```python
from build123d import *

# Parameters (mm, degrees)
RESSALTO_EXTRUS_O1_DEPTH = 59
ESBO_O2_W                = 50
ESBO_O2_H                = 43.8
CORTE_EXTRUS_O1_DEPTH    = 49
ESBO_O3_R                = 1.75
CORTE_EXTRUS_O2_DEPTH    = 92.553263186
ESBO_O4_W                = 5.65
ESBO_O4_H                = 50
ESBO_O4_R                = 1.75
RESSALTO_EXTRUS_O2_DEPTH = 1
ESBO_O5_R                = 4.35
CORTE_EXTRUS_O3_DEPTH    = 4
ESBO_O6_R                = 11.5
ESBO_O6_R_2              = 1.6
ESBO_O6_R_3              = 4.1
CORTE_EXTRUS_O4_DEPTH    = 6.2
ESBO_O7_W                = 146.645029728
ESBO_O7_H                = 95.479941405
CORTE_EXTRUS_O5_DEPTH    = 139


with BuildPart() as part:
    # Esboço1 → Ressalto-extrusão1 (new body)
    with BuildSketch(Plane.XY):
        Polygon((9, 0), (58, 43.8), (58, 50), (0, 50), (0, 0), align=None)
    extrude(amount=RESSALTO_EXTRUS_O1_DEPTH)

    # Esboço2 → Corte-extrusão1 (cut)
    with BuildSketch(Plane(origin=(58, 0, 0), x_dir=(0, 0, -1), z_dir=(1, 0, 0))):
        with Locations((-29, 21.9)):
            Rectangle(ESBO_O2_W, ESBO_O2_H)
    extrude(amount=-CORTE_EXTRUS_O1_DEPTH, mode=Mode.SUBTRACT)

    # Esboço3 → Corte-extrusão2 (cut, through all)
    with BuildSketch(Plane(origin=(9, 0, 0), x_dir=(0, 0, -1), z_dir=(1, 0, 0))):
        with Locations((-29, 11.9)):
            Circle(ESBO_O3_R)
        with Locations((-29, 31.9)):
            Circle(ESBO_O3_R)
        with Locations((-9, 31.9)):
            Circle(ESBO_O3_R)
        with Locations((-9, 11.9)):
            Circle(ESBO_O3_R)
    extrude(amount=-CORTE_EXTRUS_O2_DEPTH, mode=Mode.SUBTRACT)

    # Esboço4 → Ressalto-extrusão2 (add)
    # profile 1 of 2: a face of its own
    with BuildSketch(Plane.ZY):
        with Locations((9, 25)):
            Rectangle(ESBO_O4_W, ESBO_O4_H)
        with Locations(Location((9, 11.9, 0), (0, 0, 180))):
            Circle(ESBO_O4_R, mode=Mode.SUBTRACT)
        with Locations(Location((9, 31.9, 0), (0, 0, 180))):
            Circle(ESBO_O4_R, mode=Mode.SUBTRACT)
    # profile 2 of 2: a face of its own
    with BuildSketch(Plane.ZY):
        with Locations((29, 25)):
            Rectangle(ESBO_O4_W, ESBO_O4_H)
        with Locations(Location((29, 11.9, 0), (0, 0, 180))):
            Circle(ESBO_O4_R, mode=Mode.SUBTRACT)
        with Locations(Location((29, 31.9, 0), (0, 0, 180))):
            Circle(ESBO_O4_R, mode=Mode.SUBTRACT)
    extrude(amount=RESSALTO_EXTRUS_O2_DEPTH)

    # Esboço5 → Corte-extrusão3 (cut)
    with BuildSketch(Plane(origin=(9, 0, 0), x_dir=(0, 0, -1), z_dir=(1, 0, 0))):
        with Locations((-29, 31.9)):
            Circle(ESBO_O5_R)
        with Locations((-9, 31.9)):
            Circle(ESBO_O5_R)
        with Locations((-29, 11.9)):
            Circle(ESBO_O5_R)
        with Locations((-9, 11.9)):
            Circle(ESBO_O5_R)
    extrude(amount=-CORTE_EXTRUS_O3_DEPTH, mode=Mode.SUBTRACT)

    # Esboço6 → Corte-extrusão4 (cut)
    with BuildSketch(Plane(origin=(0, 50, 0), x_dir=(1, 0, 0), z_dir=(0, 1, 0))):
        with Locations(Location((37, -29, 0), (0, 0, 270))):
            Circle(ESBO_O6_R)
        with Locations(Location((21.5, -13.5, 0), (0, 0, 270))):
            Circle(ESBO_O6_R_2)
        with Locations(Location((52.5, -13.5, 0), (0, 0, 270))):
            Circle(ESBO_O6_R_2)
        with Locations(Location((52.5, -44.5, 0), (0, 0, 270))):
            Circle(ESBO_O6_R_2)
        with Locations(Location((21.5, -44.5, 0), (0, 0, 270))):
            Circle(ESBO_O6_R_2)
        with Locations(Location((37, -46, 0), (0, 0, 270))):
            Circle(ESBO_O6_R_3)
    extrude(amount=-CORTE_EXTRUS_O4_DEPTH, mode=Mode.SUBTRACT)


with BuildPart() as body_2:
    # Espelhar2: mirrored copy
    add(part.part.mirror(Plane(origin=(0, 0, -10), x_dir=(1, 0, 0), z_dir=(0, 0, -1))))


with BuildPart() as part_1:
    add(part.part)

    # Esboço7 → Corte-extrusão5 (cut)
    with BuildSketch(Plane(origin=(0, 0, -10), x_dir=(-1, 0, 0), z_dir=(0, 0, -1))):
        with Locations((-17.98187812, 24.060524641)):
            Rectangle(ESBO_O7_W, ESBO_O7_H)
    extrude(amount=-CORTE_EXTRUS_O5_DEPTH, mode=Mode.SUBTRACT)


solid = body_2.part
```
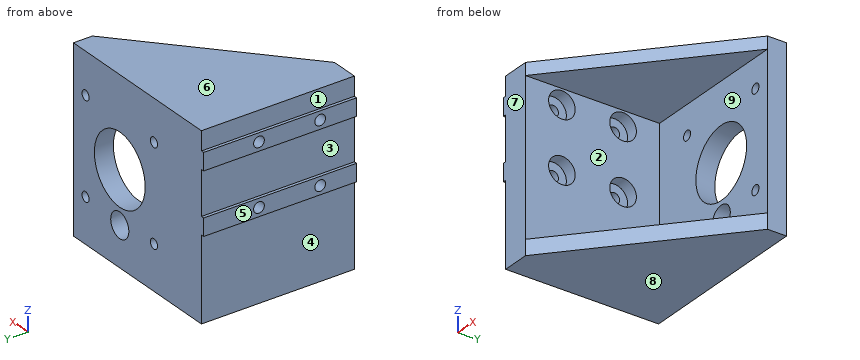
Geometry check sheet. Reference: the model listing, model coordinates, mm. Face numbers are marked on the shaded views. A direction names the side the tool comes from. Coordinates: 2 decimals unless noted, no trailing zeros. Write each loop counter-clockwise with the first axis right and the second up, starting at its lowest first coordinate (ties: lowest second). Pieces come first, ordered by that corner, then holes. Notation, with made-up numbers: M 30.25,36.5 L 37.25,36.5 A37 ccw 37.25,72.5 Z; hole C 57,43 d4. An arc over 180 degrees is marked long. One line per item, written item: value. Start each with the question number.
(1) Sectioned sample at D-D, the plane z = -43.5. Enter the section's corners in (x, y).
(2) Depth check by flat-ended pin: pin 1 (4.5 mm diameter, centred on y = 34, z = -48.5, fed in from +X); pin 2 (7 mm diameter, centred on y = 37, z = -23.5, fed in from -X); pin 3 (4.5 mm diameter, centred on y = 11.5, z = -27, fed in from +X); pin 4 (12 mm diameter, centred on x = 35, z = -54.5, fed in from -Y). Enter the tip coordinate at first touch or a pass-through.
(3) Release check for a two-part mould opening along Z. For the marked faces 6, 7, 8 and 9 record: released by +Z, released by -Z, zero draft, split by the parting line, or undercut.
(4) Scan lines: line 1 along X through (y, z) = (48.75, -33.5); line 2 along Y through (x, z) = (6.7, -49); line 3 along Y through (x, z) = (2.5, -49). Record each from-to range of solid material in increasing order. Write a range as [from, to].
(5) Sectioned sample at B-B, the plane y = 11.9. State how many separate pieces and enclosed holes the cut face has, and give its area (3 significant figures).
(6) Sectioned sample at C-C, the plane z = -64.5. Enter the section's corners in (x, y).
(7) Sectioned sample at A-A, the plane x = 21.5. Enter the section's corners in (y, z), and give its area (3 significant figures).
(8) Tool access check on the marked faces 1, 2, 3, 4 and 5. Record the directions out of +Z, -Z, +X, -X, +Y, -Y that give a thin tool (end or side, any length) a straight path to the whole face; none if there is none.
Filled sheet:
1. outline: M 0,0 L 9,0 L 9,43.8 L 26.9,43.8 L 26.9,50 L 0,50 Z; M 47.1,43.8 L 58,43.8 L 58,50 L 47.1,50 Z
2. pin 1: x = 9
2. pin 2: x = -1
2. pin 3: x = 5
2. pin 4: y = 43.8
3. face 6: released by +Z
3. face 7: zero draft
3. face 8: released by -Z
3. face 9: undercut
4. line 1: [0, 19.9], [23.1, 50.9], [54.1, 58]
4. line 2: [0, 7.55], [16.25, 27.55], [36.25, 50]
4. line 3: [0, 10.15], [13.65, 30.15], [33.65, 50]
5. separate pieces: 3
5. enclosed holes: 0
5. area: 551 mm²
6. outline: M 0,0 L 9,0 L 9,43.8 L 19.9,43.8 L 19.9,50 L 0,50 Z; M 23.1,43.8 L 33.18,43.8 L 33.18,50 L 23.1,50 Z; M 40.82,43.8 L 50.9,43.8 L 50.9,50 L 40.82,50 Z; M 54.1,43.8 L 58,43.8 L 58,50 L 54.1,50 Z
7. outline: M 11.17,-79 L 50,-79 L 50,-66.1 L 43.8,-66.1 L 43.8,-74 L 11.17,-74 Z; M 11.17,-24 L 43.8,-24 L 43.8,-31.9 L 50,-31.9 L 50,-20 L 11.17,-20 Z; M 43.8,-62.9 L 50,-62.9 L 50,-35.1 L 43.8,-35.1 Z
7. area: 620 mm²
8. face 1: +Z, -X, +Y, -Y
8. face 2: +X, -Y
8. face 3: -X, +Y, -Y
8. face 4: -Z, -X, +Y, -Y
8. face 5: +Z, -Z, -X, +Y, -Y
